Geometry check sheet. Reference: the model listing, model coordinates, mm. Coordinates: 2 decimals unless noted, no trailing zeros. Order: outer loops, then holes, each group sorted by start corner. A loop starts at its lowest first (then second) coordinate and runs counter-clockwise, first axis right, second up. Notation, with made-up numbers: M 46.5,53 L 71.5,53 A8 ccw 71.5,64 Z; hole C 8,4.5 d10. An arc over 180 degrees is marked long. Use CSV: the item, a comma, the result in double quotes. Start each with the question number.
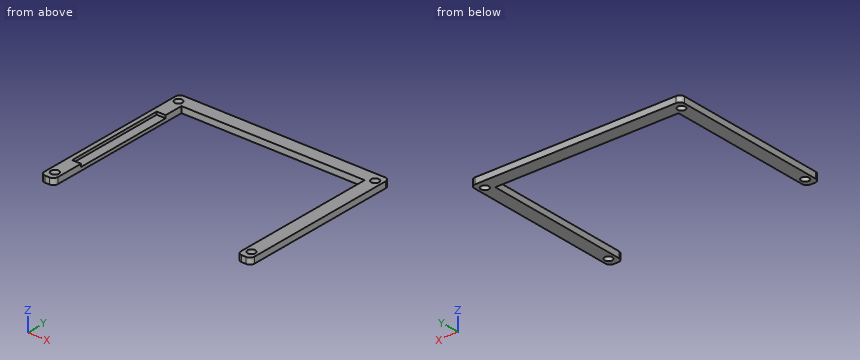
```python
from build123d import *

# Parameters (mm, degrees)
SKETCH1_R           = 1.75
BOSS_EXTRUDE1_DEPTH = 2.75
SKETCH2_W           = 4
SKETCH2_H           = 45
CUT_EXTRUDE1_DEPTH  = 1.25


with BuildPart() as part:
    # Sketch1 → Boss-Extrude1 (new body)
    with BuildSketch(Plane.XY):
        with BuildLine():
            Line((-41.592117096, -107.975551573), (-41.592117096, -113.323938617))
            ThreePointArc((-41.592117096, -113.323938617), (-42.177903534, -114.73815218), (-43.592117096, -115.323938617))
            Line((-43.592117096, -115.323938617), (-45.592117096, -115.323938617))
            ThreePointArc((-45.592117096, -115.323938617), (-47.006330659, -114.73815218), (-47.592117096, -113.323938617))
            Line((-47.592117096, -113.323938617), (-47.592117096, -43.523080591))
            ThreePointArc((-47.592117096, -43.523080591), (-47.006330659, -42.108867028), (-45.592117096, -41.523080591))
            Line((-45.592117096, -41.523080591), (44.207882904, -41.523080591))
            ThreePointArc((44.207882904, -41.523080591), (45.622096466, -42.108867028), (46.207882904, -43.523080591))
            Line((46.207882904, -43.523080591), (46.207882904, -113.323938617))
            ThreePointArc((46.207882904, -113.323938617), (45.622096466, -114.73815218), (44.207882904, -115.323938617))
            Line((44.207882904, -115.323938617), (42.207882904, -115.323938617))
            ThreePointArc((42.207882904, -115.323938617), (40.793669341, -114.73815218), (40.207882904, -113.323938617))
            Line((40.207882904, -113.323938617), (40.207882904, -107.975551573))
            Line((40.207882904, -107.975551573), (40.207882904, -47.523080591))
            Line((40.207882904, -47.523080591), (-41.592117096, -47.523080591))
            Line((-41.592117096, -47.523080591), (-41.592117096, -107.975551573))
        make_face()
        with Locations((-44.592117096, -45.523938617)):
            Circle(SKETCH1_R, mode=Mode.SUBTRACT)
        with Locations((43.207882904, -45.523938617)):
            Circle(SKETCH1_R, mode=Mode.SUBTRACT)
        with Locations((43.207882904, -111.323938617)):
            Circle(SKETCH1_R, mode=Mode.SUBTRACT)
        with Locations((-44.592117096, -111.323938617)):
            Circle(SKETCH1_R, mode=Mode.SUBTRACT)
    extrude(amount=BOSS_EXTRUDE1_DEPTH)

    # Sketch2 → Cut-Extrude1 (cut)
    with BuildSketch(Plane.XY.offset(2.75)):
        with Locations((-43.592117096, -78.423509604)):
            Rectangle(SKETCH2_W, SKETCH2_H)
    extrude(amount=-CUT_EXTRUDE1_DEPTH, mode=Mode.SUBTRACT)


solid = part.part
```
1) Section check B-B on z = 0.7. Record the boundary of the cut face in (x, y), then the cut area to 3 significant figures.
2) Section check A-A on y = -96. Record the boundary of the cut face in (x, z), then the cut area to 3 significant figures.
3) Material ranges on line 1 along X through (y, z) = (-102, 2.45); line 2 along X through (y, z) = (-70, 2.2); line 3 along Y through (x, z) = (-22, 1.9), recorded low to high.
4) Section check C-C on x = -28. Record the boundary of the cut face in (y, z).
5) Gauge pin test, flat end, axial feed: P1, Ø1.2, axis at x = -43.5, y = -88, coming from the +Z side. Record the tip position at first contact, or that the pin passes through.
Results are:
1,outline,"M -47.59,-113.32 A2 ccw -45.59,-115.32 L -43.59,-115.32 A2 ccw -41.59,-113.32 L -41.59,-47.52 L 40.21,-47.52 L 40.21,-113.32 A2 ccw 42.21,-115.32 L 44.21,-115.32 A2 ccw 46.21,-113.32 L 46.21,-43.52 A2 ccw 44.21,-41.52 L -45.59,-41.52 A2 ccw -47.59,-43.52 Z; hole C -44.59,-111.32 d3.5; hole C -44.59,-45.52 d3.5; hole C 43.21,-111.32 d3.5; hole C 43.21,-45.52 d3.5"
1,area,"1,330 mm²"
2,outline,"M -47.59,0 L -41.59,0 L -41.59,1.5 L -45.59,1.5 L -45.59,2.75 L -47.59,2.75 Z; M 40.21,0 L 46.21,0 L 46.21,2.75 L 40.21,2.75 Z"
2,area,"28.0 mm²"
3,line 1,"x = -47.59 to -41.59, 40.21 to 46.21"
3,line 2,"x = -47.59 to -45.59, 40.21 to 46.21"
3,line 3,"y = -47.52 to -41.52"
4,outline,"M -47.52,0 L -41.52,0 L -41.52,2.75 L -47.52,2.75 Z"
5,P1,"stops at z = 1.5"
